Input: dimensioned drawing with shaded views. Units: mm. Origin: part minimum x, y, z. Give positions to 0.01 mm unless a question says otherwise; leave off trailing zeros. Loops run counter-clockwise (first coordinate to the right, second up) from the corner with the lowest first, then second, coordinate; pieces in that order, holes last. Notation, with made-up numbers: (43.5, -10) -> (93.5, -10) arc R16 ccw to (93.5, 10) -> close; hole circle Ø5 at (-3, 58). An arc over 180 degrees is marked (long way). Answer as a JSON object with one key per item and string values.
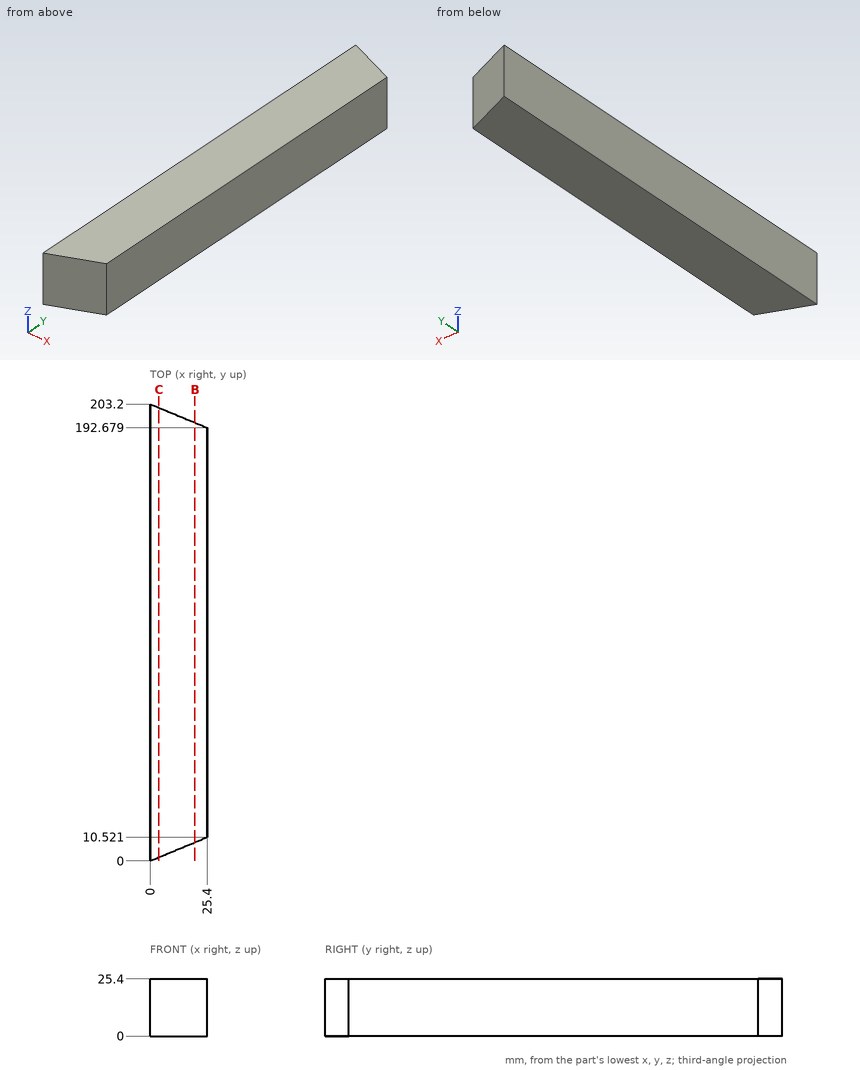
Q1. Pin query (flat end, axial travel): pin 1 (4 mm diameter, centred on x = 9.5, y = 165, fed in from -Z); pin 2 (5 mm diameter, centred on x = 22, z = 22, fed in from -Y); pin 3 (10 mm diameter, centred on x = 17.5, z = 19.5, fed in from -Y); pin 4 (12 mm diameter, centred on x = 11.5, z = 10, fed in from -Y). Return the tip coordinate at first contact, or that it passes through.
Evaluation:
{"pin 1": "stops at z = 0", "pin 2": "stops at y = 8.08", "pin 3": "stops at y = 5.18", "pin 4": "stops at y = 2.28"}
Q2. Section C-C, the plane x = 4. Return the cut outline in (y, z), then the cut area to 3 significant figures.
Evaluation:
{"outline": "(1.66, 0) -> (201.54, 0) -> (201.54, 25.4) -> (1.66, 25.4) -> close", "area": "5,080 mm2"}
Q3. Ray query, line 1 along Y through (x, z) = (15, 23); line 2 along Y through (x, z) = (4.75, 4.5); line 3 along X through (y, z) = (193.5, 20). Return the intervals inside material, ascending.
Evaluation:
{"line 1": "y = 6.21 to 196.99", "line 2": "y = 1.97 to 201.23", "line 3": "x = 0 to 23.42"}
Q4. Section B-B, the plane x = 20. Return the cut outline in (y, z), then the cut area to 3 significant figures.
Evaluation:
{"outline": "(8.28, 0) -> (194.92, 0) -> (194.92, 25.4) -> (8.28, 25.4) -> close", "area": "4,740 mm2"}
